The drawing under review shows one solid part. Ordinate dimensions are in mm from its lowest x, y, z. A direction names the side the tool comes from. Coordinates: 2 decimals unless noted, no trailing zeros. Loops run counter-clockwise (first coordinate to the right, second up) from the corner with the lowest first, then second, coordinate; pieces in that order, holes last. Notation, with made-up numbers: M 44,43.5 L 100,43.5 A17 ccw 100,72.5 Z; hole C -14,-30 d1. An arc over 180 degrees is marked long. Answer as CSV lines item,"result". Start each with the question number.
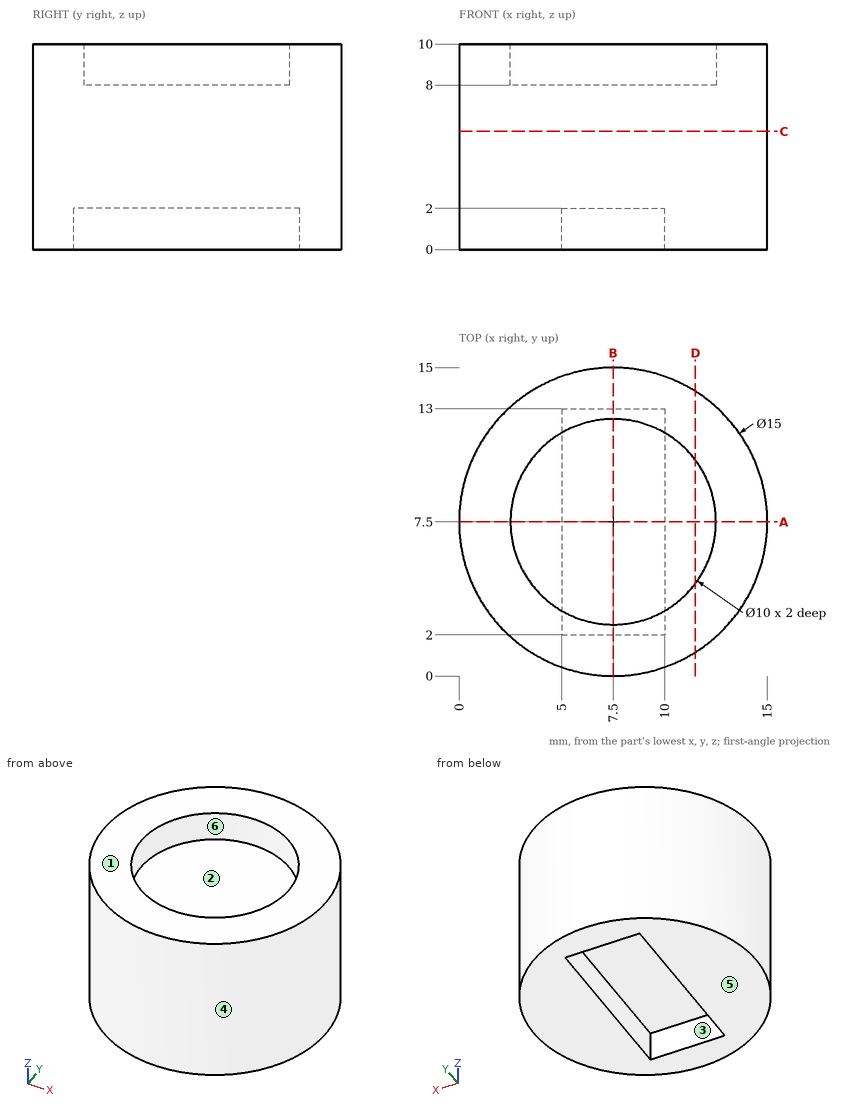
Item 1: Mouldability with a two-part tool opening along Y and no side actions: class the marked faces 4, 5 and 6 as released by +Y, released by -Y, zero draft, split by the parting line, or undercut.
Item 2: For the marked faces 1, 2 and 3, list the 3-axis set-ups (+Z, -Z, +X, -X, +Y, -Y) from which the entire face can be reached by the end or side of a thin tool; tool diameter is ignored.
Item 3: Add section C-C (z = 5.75). Give the boundary of the cut face in (x, y).
Item 4: For pin 1 (2.5 mm diameter, centred on x = 7, y = 9.5, fed in from -Z); pin 2 (2 mm diameter, centred on y = 9.5, z = 9, fed in from +X); pin 3 (1.5 mm diameter, centred on y = 3.5, z = 8, fed in from +X), all flat-tipped, find the tip position at first contact; note any pin that passes through.
Item 5: For line 1 along Y through (x, z) = (7.5, 8.65); line 2 along Z through (x, y) = (7.25, 12); line 3 along Z through (x, y) = (12.25, 8), list the stretches that pass through material, from the lowest coordinate up. Write a range as from..to.
Item 6: Add section B-B (x = 7.5). Give the boundary of the cut face in (y, z).
Item 7: Add section A-A (y = 7.5). Give the boundary of the cut face in (x, z), plus the area to 3 significant figures.
Item 8: Add section D-D (x = 11.5). Give the boundary of the cut face in (y, z), plus the area to 3 significant figures.
Response:
1,face 4,"split by the parting line"
1,face 5,"zero draft"
1,face 6,"undercut"
2,face 1,"+Z, +X, -X, +Y, -Y"
2,face 2,"+Z"
2,face 3,"-Z"
3,outline,"C 7.5,7.5 d15"
4,pin 1,"z = 2"
4,pin 2,"x = 14.93"
4,pin 3,"x = 14.26"
5,line 1,"0..2.5, 12.5..15"
5,line 2,"2..8"
5,line 3,"0..8"
6,outline,"M 0,0 L 2,0 L 2,2 L 13,2 L 13,0 L 15,0 L 15,10 L 12.5,10 L 12.5,8 L 2.5,8 L 2.5,10 L 0,10 Z"
7,outline,"M 0,0 L 5,0 L 5,2 L 10,2 L 10,0 L 15,0 L 15,10 L 12.5,10 L 12.5,8 L 2.5,8 L 2.5,10 L 0,10 Z"
7,area,"120 mm²"
8,outline,"M 1.16,0 L 13.84,0 L 13.84,10 L 10.5,10 L 10.5,8 L 4.5,8 L 4.5,10 L 1.16,10 Z"
8,area,"115 mm²"
